Geometry: see drawing. Coordinates: mm, zero at the bounding-box minimum. A direction names the side the tool comes from. Give positions to 0.01 mm unless a question says otherwise; leave off trailing zeros. Loops run counter-clockwise (first coordinate to the right, second up) from the corner with the lowest first, then second, coordinate; pieces in that order, holes last. Notation, with made-up numbers: M 89,82.25 L 113,82.25 A21 cw 113,93.25 Z; hole C 74,86.5 d4. An arc over 180 degrees is marked long. Answer in a Markdown table with one row per item.
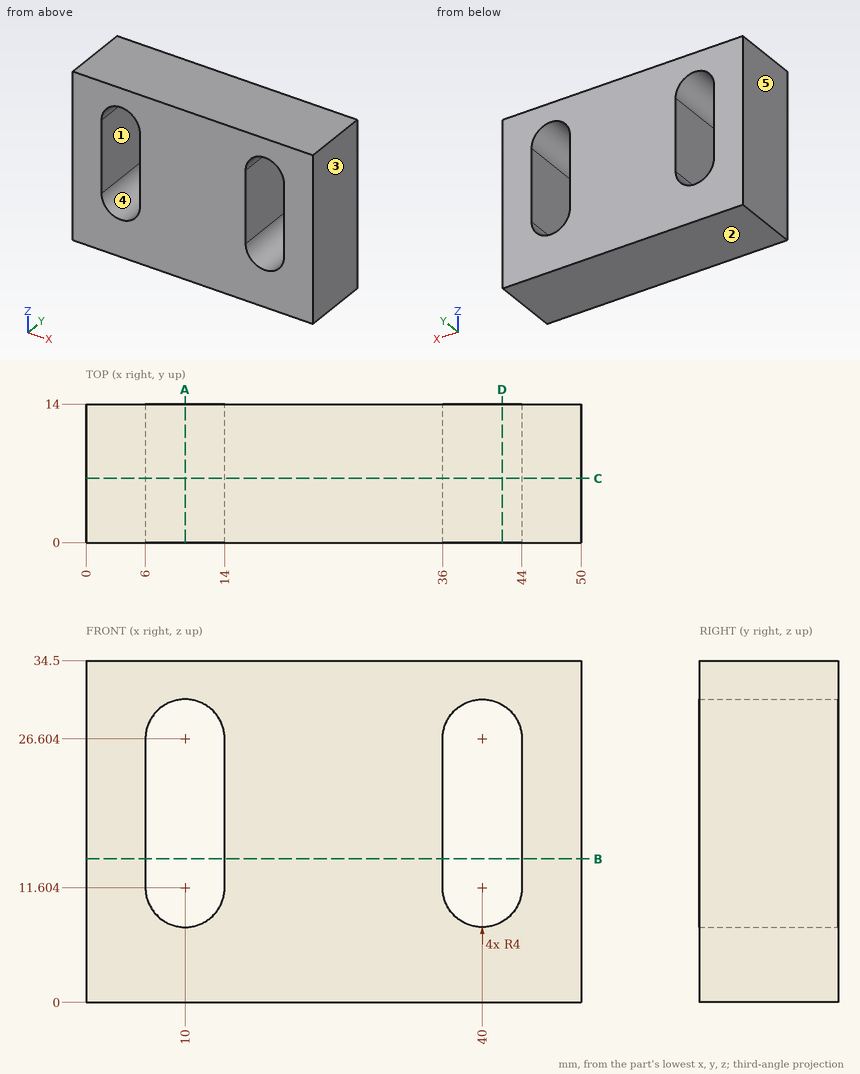
1) Material intervals for L1, parallel to X at y = 8.25, z = 14.5; L2, parallel to X at y = 8.75, z = 28.5; L3, parallel to Z at x = 9, y = 0.5, sorted ascending.
Reply:
| item | result |
|---|---|
| L1 | x = 0 to 6, 14 to 36, 44 to 50 |
| L2 | x = 0 to 6.48, 13.52 to 36.48, 43.52 to 50 |
| L3 | z = 0 to 7.73, 30.48 to 34.5 |
2) Section C-C, the plane y = 6.5. Return loops of the section in (x, z).
Reply:
| item | result |
|---|---|
| outline | M 0,0 L 50,0 L 50,34.5 L 0,34.5 Z; hole M 6,11.6 A4 ccw 14,11.6 L 14,26.6 A4 ccw 6,26.6 Z; hole M 36,11.6 A4 ccw 44,11.6 L 44,26.6 A4 ccw 36,26.6 Z |
3) Set-up query: the marked faces 1 and 2. Return all of +Z, -Z, +X, -X, +Y, -Y with unobstructed straight access to the full face (end or side cutting, diameter ignored); none if empty.
Reply:
| item | result |
|---|---|
| face 1 | +Y, -Y |
| face 2 | -Z, +X, -X, +Y, -Y |
4) Section B-B, the plane z = 14.5. Return loops of the section in (x, y).
Reply:
| item | result |
|---|---|
| outline | M 0,0 L 6,0 L 6,14 L 0,14 Z; M 14,0 L 36,0 L 36,14 L 14,14 Z; M 44,0 L 50,0 L 50,14 L 44,14 Z |
5) Section A-A, the plane x = 10. Return loops of the section in (y, z).
Reply:
| item | result |
|---|---|
| outline | M 0,0 L 14,0 L 14,7.6 L 0,7.6 Z; M 0,30.6 L 14,30.6 L 14,34.5 L 0,34.5 Z |
6) Pull-direction query (X, two-part tool) for the marked faces 3, 4 and 5; classes: released by +X, released by -X, zero draft, split by the parting line, or undercut.
Reply:
| item | result |
|---|---|
| face 3 | released by +X |
| face 4 | undercut |
| face 5 | released by -X |
7) Section D-D, the plane x = 42. Return loops of the section in (y, z), then the cut area to 3 significant figures.
Reply:
| item | result |
|---|---|
| outline | M 0,0 L 14,0 L 14,8.14 L 0,8.14 Z; M 0,30.07 L 14,30.07 L 14,34.5 L 0,34.5 Z |
| area | 176 mm² |
